from build123d import *

# Parameters (mm, degrees)
SKETCH1_W           = 74
SKETCH1_H           = 59
BOSS_EXTRUDE1_DEPTH = 2
SKETCH2_W           = 74
SKETCH2_H           = 59
SKETCH2_W_2         = 69
SKETCH2_H_2         = 54
BOSS_EXTRUDE2_DEPTH = 2
SKETCH3_W           = 2.5
SKETCH3_H           = 18
BOSS_EXTRUDE3_DEPTH = 11
SKETCH4_W           = 30
SKETCH4_H           = 4
BOSS_EXTRUDE4_DEPTH = 100
SKETCH5_W           = 4
SKETCH5_H           = 30
BOSS_EXTRUDE5_DEPTH = 30
SKETCH6_W           = 68
SKETCH6_H           = 30
SKETCH6_W_2         = 41
SKETCH6_H_2         = 21
BOSS_EXTRUDE6_DEPTH = 4
SKETCH7_R           = 1.75
SKETCH7_W           = 9.5
SKETCH7_H           = 6.4
CUT_EXTRUDE1_DEPTH  = 5
CUT_EXTRUDE2_DEPTH  = 2.5
SKETCH9_R           = 4
CUT_EXTRUDE3_DEPTH  = 10
SKETCH10_RX         = 12.5
SKETCH10_RY         = 4
CUT_EXTRUDE4_DEPTH  = 2


with BuildPart() as part:
    # Sketch1 → Boss-Extrude1 (new body)
    with BuildSketch(Plane(origin=(0, 0, 0), x_dir=(1, 0, 0), z_dir=(0, 1, 0))):
        Rectangle(SKETCH1_W, SKETCH1_H)
    extrude(amount=BOSS_EXTRUDE1_DEPTH)

    # Sketch2 → Boss-Extrude2 (add)
    with BuildSketch(Plane(origin=(0, 2, 0), x_dir=(1, 0, 0), z_dir=(0, 1, 0))):
        Rectangle(SKETCH2_W, SKETCH2_H)
        Rectangle(SKETCH2_W_2, SKETCH2_H_2, mode=Mode.SUBTRACT)
    extrude(amount=BOSS_EXTRUDE2_DEPTH)

    # Sketch3 → Boss-Extrude3 (add)
    with BuildSketch(Plane(origin=(0, 4, 0), x_dir=(1, 0, 0), z_dir=(0, 1, 0))):
        Polygon((22.5, -27), (22.5, -29.5), (-37, -29.5), (-37, 29.5), (37, 29.5), (37, 24.5), (34.5, 24.5), (34.5, 27), (-34.5, 27), (-34.5, -27), align=None)
        with Locations((35.75, 4.5)):
            Rectangle(SKETCH3_W, SKETCH3_H)
    extrude(amount=BOSS_EXTRUDE3_DEPTH)

    # Sketch4 → Boss-Extrude4 (add)
    with BuildSketch(Plane.ZY.offset(37)):
        with Locations((0, 2)):
            Rectangle(SKETCH4_W, SKETCH4_H)
    extrude(amount=BOSS_EXTRUDE4_DEPTH)

    # Sketch5 → Boss-Extrude5 (add)
    with BuildSketch(Plane(origin=(0, 4, 0), x_dir=(1, 0, 0), z_dir=(0, 1, 0))):
        with Locations((-71, 0)):
            Rectangle(SKETCH5_W, SKETCH5_H)
        with Locations((-135, 0)):
            Rectangle(SKETCH5_W, SKETCH5_H)
    extrude(amount=BOSS_EXTRUDE5_DEPTH)

    # Sketch6 → Boss-Extrude6 (add)
    with BuildSketch(Plane(origin=(0, 34, 0), x_dir=(1, 0, 0), z_dir=(0, 1, 0))):
        with Locations((-103, 0)):
            Rectangle(SKETCH6_W, SKETCH6_H)
        with Locations((-103, 0)):
            Rectangle(SKETCH6_W_2, SKETCH6_H_2, mode=Mode.SUBTRACT)
    extrude(amount=BOSS_EXTRUDE6_DEPTH)

    # Sketch7 → Cut-Extrude1 (cut)
    with BuildSketch(Plane(origin=(0, 38, 0), x_dir=(1, 0, 0), z_dir=(0, 1, 0))):
        with Locations((-128.25, 5)):
            Circle(SKETCH7_R)
        with Locations((-77.75, 5)):
            Circle(SKETCH7_R)
        with Locations((-77.75, -5)):
            Circle(SKETCH7_R)
        with Locations((-128.25, -5)):
            Circle(SKETCH7_R)
        with Locations((-77.75, 0)):
            Rectangle(SKETCH7_W, SKETCH7_H)
    extrude(amount=-CUT_EXTRUDE1_DEPTH, mode=Mode.SUBTRACT)

    # Sketch8 → Cut-Extrude2 (cut)
    with BuildSketch(Plane.XZ.offset(-34)):
        Polygon((-131.25, 6.732050808), (-131.25, 3.267949192), (-128.25, 1.535898385), (-125.25, 3.267949192), (-125.25, 6.732050808), (-128.25, 8.464101615), align=None)
        Polygon((-128.25, -1.535898385), (-131.25, -3.267949192), (-131.25, -6.732050808), (-128.25, -8.464101615), (-125.25, -6.732050808), (-125.25, -3.267949192), align=None)
        Polygon((-74.75, 3.267949192), (-74.75, 6.732050808), (-77.75, 8.464101615), (-80.75, 6.732050808), (-80.75, 3.267949192), (-77.75, 1.535898385), align=None)
        Polygon((-74.75, -6.732050808), (-74.75, -3.267949192), (-77.75, -1.535898385), (-80.75, -3.267949192), (-80.75, -6.732050808), (-77.75, -8.464101615), align=None)
    extrude(amount=-CUT_EXTRUDE2_DEPTH, mode=Mode.SUBTRACT)

    # Sketch9 → Cut-Extrude3 (cut)
    with BuildSketch(Plane(origin=(0, 4, 0), x_dir=(1, 0, 0), z_dir=(0, 1, 0))):
        with Locations((-64, 0)):
            Circle(SKETCH9_R)
    extrude(amount=-CUT_EXTRUDE3_DEPTH, mode=Mode.SUBTRACT)

    # Sketch10 → Cut-Extrude4 (cut)
    with BuildSketch(Plane.XZ):
        with Locations(Location((-64, 0), (0, 0, 90))):
            Ellipse(SKETCH10_RX, SKETCH10_RY)
        with Locations((-64, 0)):
            Ellipse(SKETCH10_RX, SKETCH10_RY)
    extrude(amount=-CUT_EXTRUDE4_DEPTH, mode=Mode.SUBTRACT)


solid = part.part
Design review of the part built by this model. Coordinates are the model's own, in mm. A direction names the side the tool comes from. Coordinates: 2 decimals unless noted, no trailing zeros. Order: outer loops, then holes, each group sorted by start corner. A loop starts at its lowest first (then second) coordinate and runs counter-clockwise, first axis right, second up.
Item 1: For line 1 (X direction, y = 37.35, z = -5); line 2 (X direction, y = 12.5, z = 7); line 3 (X direction, y = 2.5, z = 0), list the stretches that pass through material, from the lowest coordinate up.
Item 2: For pin 1 Ø10 at (x, z) = (-26, -23.5) entering from -Y; pin 2 Ø9 at (x, z) = (-64, 0) entering from -Y; pin 3 Ø3 at (x, y) = (-101.5, 37) entering from -Z; pin 4 Ø5 at (x, z) = (-25, 9) entering from +Y, all flat-tipped, find the tip position at first contact; note any pin that passes through.
Item 3: Take a section at A-A, the plane y = 24. Write out the cut boundary in (x, z).
Item 4: Take a section at C-C, the plane z = -19. Write out the cut boundary in (x, y).
Item 5: The part is to be moulded in two halves that separate along Y. For faces 5 (the flat face through (-77, 37, 3.2)), 6 (the flat face through (-67, 2, -3)), 7 (the flat face through (-78, 36.5, -7)), say which applies: pulls with the +Y half, pulls with the -Y half, needs draft (parallel to the pull), parting line crosses it, or undercut.
Item 6: For faces 1 (the flat face through (35, 4, 20)), 2 (the flat face through (-69, 21, 0)), 3 (the flat face through (-82.5, 36, -7)), 4 (the flat face through (-130, 36.5, 4)), list the 3-axis set-ups (+Z, -Z, +X, -X, +Y, -Y) from which the entire face can be reached by the end or side of a thin tool; tool diameter is ignored.
Item 7: Take a section at B-B, the plane x = -7.5. Write out the cut boundary in (y, z), then the cut area to 3 significant figures.
The answers:
1. line 1: x = -137 to -130, -126.5 to -123.5, -82.5 to -79.5, -76 to -69
1. line 2: x = -137 to -133, -73 to -69, -37 to -34.5
1. line 3: x = -137 to -68, -60 to -34.5, 34.5 to 37
2. pin 1: stops at y = 0
2. pin 2: stops at y = 2
2. pin 3: stops at z = -15
2. pin 4: stops at y = 2
3. outline: (-137, -15) - (-133, -15) - (-133, 15) - (-137, 15) - close; (-73, -15) - (-69, -15) - (-69, 15) - (-73, 15) - close
4. outline: (-37, 0) - (37, 0) - (37, 4) - (34.5, 4) - (34.5, 2) - (-34.5, 2) - (-34.5, 15) - (-37, 15) - close
5. face 5: needs draft
5. face 6: pulls with the -Y half
5. face 7: undercut
6. face 1: +Z, +X, +Y
6. face 2: +Z, -Z, +Y
6. face 3: +Y
6. face 4: none
7. outline: (0, -29.5) - (15, -29.5) - (15, -27) - (2, -27) - (2, 27) - (15, 27) - (15, 29.5) - (0, 29.5) - close
7. area: 183 mm2
